from build123d import *

# Parameters (mm, degrees)
SKETCH2_W                = 110
SKETCH2_H                = 55
BOSS_EXTRUDE1_DEPTH      = 1.5875
M4_CLEARANCE_HOLE1_D     = 4.5
M4_CLEARANCE_HOLE2_D     = 4.5
CHAMFER1_SIZE            = 15
FILLET1_R                = 15
SKETCH8_R                = 11
CUT_EXTRUDE1_DEPTH       = 4.175
M4_CLEARANCE_HOLE3_D     = 4.3
M4_CLEARANCE_HOLE3_DEPTH = 3.175


with BuildPart() as part:
    # Sketch2 → Boss-Extrude1 (new body, symmetric)
    with BuildSketch(Plane(origin=(0, 0, 0), x_dir=(1, 0, 0), z_dir=(0, 1, 0))):
        Rectangle(SKETCH2_W, SKETCH2_H)
    extrude(amount=BOSS_EXTRUDE1_DEPTH, both=True)

    # M4 Clearance Hole1 (through all)
    with Locations(Plane(origin=(0, 1.5875, 0), x_dir=(1, 0, 0), z_dir=(0, 1, 0))):
        with Locations((-46, 5.5), (-21, 20.5), (21, 20.5), (46, 5.5), (0, 22.5)):
            Hole(M4_CLEARANCE_HOLE1_D / 2)

    # M4 Clearance Hole2 (through all)
    with Locations(Plane(origin=(0, -1.5875, 0), x_dir=(-1, 0, 0), z_dir=(0, -1, 0))):
        with Locations((37.5, -17), (-37.5, -17)):
            Hole(M4_CLEARANCE_HOLE2_D / 2)

    # Chamfer1
    chamfer1_edges = [part.edges().sort_by_distance(p)[0] for p in [
        (-55, 0, -27.5),
        (55, 0, -27.5),
    ]]
    chamfer(chamfer1_edges, length=CHAMFER1_SIZE)

    # Fillet1
    fillet1_edges = [part.edges().sort_by_distance(p)[0] for p in [
        (-55, 0, -12.5),
        (40, 0, -27.5),
        (-40, 0, -27.5),
        (55, 0, -12.5),
        (55, 0, 27.5),
        (-55, 0, 27.5),
    ]]
    fillet(fillet1_edges, radius=FILLET1_R)

    # Sketch8 → Cut-Extrude1 (cut, through all)
    with BuildSketch(Plane(origin=(0, -1.5875, 0), x_dir=(-1, 0, 0), z_dir=(0, -1, 0))):
        with Locations((16, -5.635528726)):
            Circle(SKETCH8_R)
    extrude(amount=-CUT_EXTRUDE1_DEPTH, mode=Mode.SUBTRACT)

    # M4 Clearance Hole3
    with Locations(Plane(origin=(0, -1.5875, 0), x_dir=(-1, 0, 0), z_dir=(0, -1, 0))):
        with Locations((16, 9.864471274), (2.576606241, -13.385528726), (29.423393759, -13.385528726)):
            Hole(M4_CLEARANCE_HOLE3_D / 2, depth=M4_CLEARANCE_HOLE3_DEPTH)


solid = part.part
Work out the finished part from the listing and answer in its coordinate system (mm). Give positions to 0.01 mm unless a question says otherwise; leave off trailing zeros. Write each loop counter-clockwise with the first axis right and the second up, starting at its lowest first coordinate (ties: lowest second). Pieces come first, ordered by that corner, then holes.
Q1. The part is cut by section D-D on z = 21.5. Give the vertices of the cut face in (x, y), and give its area (3 significant figures).
Answer:
outline: (-52, -1.59) - (52, -1.59) - (52, 1.59) - (-52, 1.59) - close
area: 330 mm2
Q2. The part is cut by section A-A on x = -16. Give the vertices of the cut face in (y, z), and give its area (3 significant figures).
Answer:
outline: (-1.59, -27.5) - (1.59, -27.5) - (1.59, -12.01) - (-1.59, -12.01) - close; (-1.59, -7.71) - (1.59, -7.71) - (1.59, -5.36) - (-1.59, -5.36) - close; (-1.59, 16.64) - (1.59, 16.64) - (1.59, 27.5) - (-1.59, 27.5) - close
area: 91.1 mm2
Q3. For a pull along Z with two mould halves and no side action, classify faces 1 (the face through (48.248, -0.022, -5.599)), 2 (the face through (-1, -1.588, 0)), 3 (the face through (50.49, 0.02, 23.22)), 4 (the face through (-53.89, -0.02, -11.95)) as released by +Z, released by -Z, zero draft, split by the parting line, or undercut.
Answer:
face 1: undercut
face 2: zero draft
face 3: released by +Z
face 4: released by -Z
Q4. The part is cut by section B-B on z = 3. Give the vertices of the cut face in (x, y).
Answer:
outline: (-55, -1.59) - (-26.68, -1.59) - (-26.68, 1.59) - (-55, 1.59) - close; (-5.32, -1.59) - (55, -1.59) - (55, 1.59) - (-5.32, 1.59) - close
Q5. Straight lines are drawn through the part: L1, parallel to Z at x = -16, y = -0.3; L2, parallel to X at y = 0.5, z = -7; L3, parallel to X at y = 0.1, z = -7.5. For each, find the intervals that lie inside material, in ascending order.
Answer:
L1: z = -27.5 to -12.01, -7.71 to -5.36, 16.64 to 27.5
L2: x = -54.98 to -47.68, -44.32 to 44.32, 47.68 to 54.98
L3: x = -54.95 to -47.03, -44.97 to 44.97, 47.03 to 54.95
Q6. The part is cut by section C-C on x = -37.5. Give the vertices of the cut face in (y, z), and give its area (3 significant figures).
Answer:
outline: (-1.59, -27.03) - (1.59, -27.03) - (1.59, 14.75) - (-1.59, 14.75) - close; (-1.59, 19.25) - (1.59, 19.25) - (1.59, 27.5) - (-1.59, 27.5) - close
area: 159 mm2
